Here's how the part is built. I have some questions about the finished solid (model axes, mm). Face numbers are marked on the shaded views. A direction names the side the tool comes from. Round coordinates to 2 decimals unless told otherwise and drop trailing zeros. Order: outer loops, then holes, each group sorted by start corner. A loop starts at its lowest first (then second) coordinate and runs counter-clockwise, first axis right, second up. Notation, with made-up numbers: (-24.75, 63.5) -> (19.25, 63.5) arc R18 ccw to (19.25, 71.5) -> close; hole circle Ø5 at (-32, 72). An arc over 180 degrees is marked (long way). One line per item, written item: value.
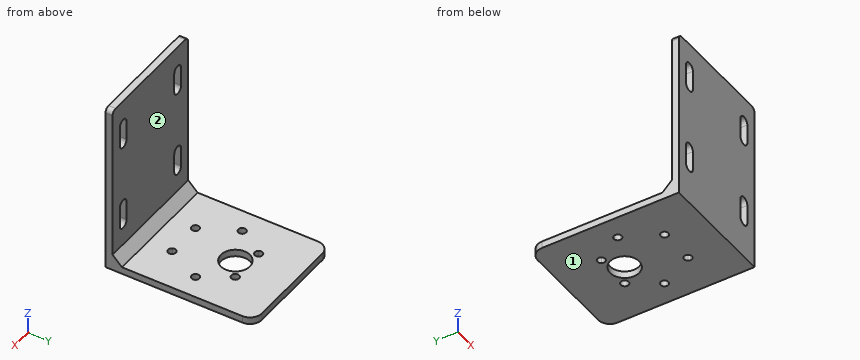
```python
from build123d import *

# Parameters (mm, degrees)
EXTRUDE_2_DEPTH     = 3
SKETCH_2_W          = 50
SKETCH_2_H          = 3
EXTRUDE_3_DEPTH     = 3
SKETCH_3_W          = 50
SKETCH_3_H          = 3
EXTRUDE_5_DEPTH     = 70
CUT_EXTRUDE_1_DEPTH = 98.744565066
FILLET_1_R          = 5
FILLET_2_R          = 2
SKETCH_5_W          = 4
SKETCH_5_H          = 4
EXTRUDE_6_DEPTH     = 4
SKETCH_6_W          = 4
SKETCH_6_H          = 4
EXTRUDE_7_DEPTH     = 46
CUT_EXTRUDE_2_DEPTH = 95.435162943


with BuildPart() as part:
    # 草图1 → 凸台-拉伸2 (new body)
    with BuildSketch(Plane.XY):
        with BuildLine():
            Line((25, 6), (25, 30))
            Line((25, 30), (-25, 30))
            Line((-25, 30), (-25, 6))
            Line((-25, 6), (-16.431676725, 6))
            ThreePointArc((-16.431676725, 6), (0, 16), (16.431676725, 6))
            Line((16.431676725, 6), (25, 6))
        make_face()
        with BuildLine():
            Line((25, -30), (25, -1))
            Line((25, -1), (18.439088915, -1))
            ThreePointArc((18.439088915, -1), (18.484765956, -1.749381895), (18.5, -2.5))
            ThreePointArc((18.5, -2.5), (-4.374013065, -20.475483574), (-16.431676725, 6))
            Line((-16.431676725, 6), (-25, 6))
            Line((-25, 6), (-25, -30))
            Line((-25, -30), (25, -30))
        make_face()
        with BuildLine():
            Line((25, -1), (25, 6))
            Line((25, 6), (16.431676725, 6))
            ThreePointArc((16.431676725, 6), (17.783210455, 2.599747633), (18.439088915, -1))
            Line((18.439088915, -1), (25, -1))
        make_face()
        with BuildLine():
            ThreePointArc((18.5, -2.5), (18.484765956, -1.749381895), (18.439088915, -1))
            Line((18.439088915, -1), (17.077248621, -1))
            ThreePointArc((17.077248621, -1), (16.619172939, -2.1409717), (15.499289324, -2.648426564))
            ThreePointArc((15.499289324, -2.648426564), (13.783292906, -9.590192993), (9.133777755, -15.022943101))
            ThreePointArc((9.133777755, -15.022943101), (9.324554056, -15.446200161), (9.389869855, -15.905847832))
            ThreePointArc((9.389869855, -15.905847832), (8.134145395, -17.508048443), (6.278297978, -16.671555119))
            ThreePointArc((6.278297978, -16.671555119), (0, -18), (-6.278297978, -16.671555119))
            ThreePointArc((-6.278297978, -16.671555119), (-8.564869855, -17.334789748), (-9.133777755, -15.022943101))
            ThreePointArc((-9.133777755, -15.022943101), (-13.783292906, -9.590192993), (-15.499289324, -2.648426564))
            ThreePointArc((-15.499289324, -2.648426564), (-17.069504119, -0.840322581), (-15.18038717, 0.631428645))
            ThreePointArc((-15.18038717, 0.631428645), (-14.324684332, 3.420592774), (-12.961481397, 6))
            Line((-12.961481397, 6), (-16.431676725, 6))
            ThreePointArc((-16.431676725, 6), (-4.374013065, -20.475483574), (18.5, -2.5))
        make_face()
        with BuildLine():
            Line((12.961481397, 6), (16.431676725, 6))
            ThreePointArc((16.431676725, 6), (0, 16), (-16.431676725, 6))
            Line((-16.431676725, 6), (-12.961481397, 6))
            ThreePointArc((-12.961481397, 6), (-11.229253628, 8.184281115), (-9.133777755, 10.022943101))
            ThreePointArc((-9.133777755, 10.022943101), (-8.564869855, 12.334789748), (-6.278297978, 11.671555119))
            ThreePointArc((-6.278297978, 11.671555119), (0, 13), (6.278297978, 11.671555119))
            ThreePointArc((6.278297978, 11.671555119), (8.134145395, 12.508048443), (9.389869855, 10.905847832))
            ThreePointArc((9.389869855, 10.905847832), (9.324554056, 10.446200161), (9.133777755, 10.022943101))
            ThreePointArc((9.133777755, 10.022943101), (11.229253628, 8.184281115), (12.961481397, 6))
        make_face()
        with BuildLine():
            ThreePointArc((15.18038717, 0.631428645), (14.324684332, 3.420592774), (12.961481397, 6))
            Line((12.961481397, 6), (6.15, 6))
            ThreePointArc((6.15, 6), (0, -0.15), (-6.15, 6))
            Line((-6.15, 6), (-12.961481397, 6))
            ThreePointArc((-12.961481397, 6), (-14.324684332, 3.420592774), (-15.18038717, 0.631428645))
            ThreePointArc((-15.18038717, 0.631428645), (-14.176284714, 0.075913242), (-13.777248621, -1))
            ThreePointArc((-13.777248621, -1), (-14.286276921, -2.191924318), (-15.499289324, -2.648426564))
            ThreePointArc((-15.499289324, -2.648426564), (-13.783292906, -9.590192993), (-9.133777755, -15.022943101))
            ThreePointArc((-9.133777755, -15.022943101), (-7.280222183, -14.321163631), (-6.089869855, -15.905847832))
            ThreePointArc((-6.089869855, -15.905847832), (-6.137669243, -16.300123373), (-6.278297978, -16.671555119))
            ThreePointArc((-6.278297978, -16.671555119), (0, -18), (6.278297978, -16.671555119))
            ThreePointArc((6.278297978, -16.671555119), (6.914869855, -14.476905916), (9.133777755, -15.022943101))
            ThreePointArc((9.133777755, -15.022943101), (13.783292906, -9.590192993), (15.499289324, -2.648426564))
            ThreePointArc((15.499289324, -2.648426564), (13.784993122, -1.159677419), (15.18038717, 0.631428645))
        make_face()
        with BuildLine():
            Line((6.15, 6), (12.961481397, 6))
            ThreePointArc((12.961481397, 6), (11.229253628, 8.184281115), (9.133777755, 10.022943101))
            ThreePointArc((9.133777755, 10.022943101), (6.914869855, 9.476905916), (6.278297978, 11.671555119))
            ThreePointArc((6.278297978, 11.671555119), (0, 13), (-6.278297978, 11.671555119))
            ThreePointArc((-6.278297978, 11.671555119), (-6.137669243, 11.300123373), (-6.089869855, 10.905847832))
            ThreePointArc((-6.089869855, 10.905847832), (-7.280222183, 9.321163631), (-9.133777755, 10.022943101))
            ThreePointArc((-9.133777755, 10.022943101), (-11.229253628, 8.184281115), (-12.961481397, 6))
            Line((-12.961481397, 6), (-6.15, 6))
            ThreePointArc((-6.15, 6), (0, 12.15), (6.15, 6))
        make_face()
        with BuildLine():
            ThreePointArc((18.439088915, -1), (17.783210455, 2.599747633), (16.431676725, 6))
            Line((16.431676725, 6), (12.961481397, 6))
            ThreePointArc((12.961481397, 6), (14.324684332, 3.420592774), (15.18038717, 0.631428645))
            ThreePointArc((15.18038717, 0.631428645), (16.503161862, 0.250963907), (17.077248621, -1))
            Line((17.077248621, -1), (18.439088915, -1))
        make_face()
    extrude(amount=EXTRUDE_2_DEPTH)

    # 草图2 → 凸台-拉伸3 (add)
    with BuildSketch(Plane.XZ.offset(30)):
        with Locations((0, 1.5)):
            Rectangle(SKETCH_2_W, SKETCH_2_H)
    extrude(amount=EXTRUDE_3_DEPTH)

    # 草图3 → 凸台-拉伸5 (add)
    with BuildSketch(Plane.XY.offset(3)):
        with Locations((0, -31.5)):
            Rectangle(SKETCH_3_W, SKETCH_3_H)
    extrude(amount=EXTRUDE_5_DEPTH)

    # 草图4 → 切除-拉伸1 (cut, through all)
    with BuildSketch(Plane(origin=(0, -30, 0), x_dir=(1, 0, 0), z_dir=(0, 1, 0))):
        with BuildLine():
            Line((-15.75, -53.85), (-15.75, -62.15))
            ThreePointArc((-15.75, -62.15), (-18, -64.4), (-20.25, -62.15))
            Line((-20.25, -62.15), (-20.25, -53.85))
            ThreePointArc((-20.25, -53.85), (-18, -51.6), (-15.75, -53.85))
        make_face()
        with BuildLine():
            Line((15.75, -53.85), (15.75, -62.15))
            ThreePointArc((15.75, -62.15), (18, -64.4), (20.25, -62.15))
            Line((20.25, -62.15), (20.25, -53.85))
            ThreePointArc((20.25, -53.85), (18, -51.6), (15.75, -53.85))
        make_face()
        with BuildLine():
            Line((-15.75, -16.85), (-15.75, -25.15))
            ThreePointArc((-15.75, -25.15), (-18, -27.4), (-20.25, -25.15))
            Line((-20.25, -25.15), (-20.25, -16.85))
            ThreePointArc((-20.25, -16.85), (-18, -14.6), (-15.75, -16.85))
        make_face()
        with BuildLine():
            Line((15.75, -16.85), (15.75, -25.15))
            ThreePointArc((15.75, -25.15), (18, -27.4), (20.25, -25.15))
            Line((20.25, -25.15), (20.25, -16.85))
            ThreePointArc((20.25, -16.85), (18, -14.6), (15.75, -16.85))
        make_face()
    extrude(amount=-CUT_EXTRUDE_1_DEPTH, mode=Mode.SUBTRACT)

    # 圆角1
    fillet_1_edges = [part.edges().sort_by_distance(p)[0] for p in [
        (-25, 30, 1.5),
        (25, 30, 1.5),
    ]]
    fillet(fillet_1_edges, radius=FILLET_1_R)

    # 圆角2
    fillet_2_edges = [part.edges().sort_by_distance(p)[0] for p in [
        (25, -31.5, 73),
        (-25, -31.5, 73),
    ]]
    fillet(fillet_2_edges, radius=FILLET_2_R)

    # 草图5 → 凸台-拉伸6 (add)
    with BuildSketch(Plane(origin=(0, -30, 0), x_dir=(1, 0, 0), z_dir=(0, 1, 0))):
        with Locations((23, -5)):
            Rectangle(SKETCH_5_W, SKETCH_5_H)
    extrude(amount=EXTRUDE_6_DEPTH)

    # 草图6 → 凸台-拉伸7 (add)
    with BuildSketch(Plane.ZY.offset(-21)):
        with Locations((5, -28)):
            Rectangle(SKETCH_6_W, SKETCH_6_H)
    extrude(amount=EXTRUDE_7_DEPTH)

    # 草图7 → 切除-拉伸2 (cut, through all)
    with BuildSketch(Plane(origin=(25, 0, 0), x_dir=(0, 0, -1), z_dir=(1, 0, 0))):
        Polygon((-7, -30), (-7, -26), (-3, -26), align=None)
    extrude(amount=-CUT_EXTRUDE_2_DEPTH, mode=Mode.SUBTRACT)


solid = part.part
```
Q1. Which directions (+Z, -Z, +X, -X, +Y, -Y) give clear straight access to the entire face, cutting with the end or side of a thin tool? Please do the marked faces 1 and 2.
Answers:
face 1: -Z, +X, -X, +Y, -Y
face 2: +Z, +X, -X, +Y
Q2. I need wall thicknesses on line 1 along Y through (x, z) = (0, 2.25); line 2 along Z through (x, y) = (14, 20.5); line 3 along Y through (x, z) = (10, 42.5). Which ranges of each line are inside material? Lowest first, please.
Answers:
line 1: -33 to -0.15, 12.15 to 30
line 2: 0 to 3
line 3: -33 to -30
Q3. I want a section at D-D on x = -18. Write out the boundary of the cut face in (y, z), then the cut area to 3 significant figures.
Answers:
outline: (-33, 0) -> (30, 0) -> (30, 3) -> (-26, 3) -> (-30, 7) -> (-30, 14.6) -> (-33, 14.6) -> close; (-33, 27.4) -> (-30, 27.4) -> (-30, 51.6) -> (-33, 51.6) -> close; (-33, 64.4) -> (-30, 64.4) -> (-30, 73) -> (-33, 73) -> close
area: 330 mm2
Q4. I want a section at A-A on x = 0. Write out the boundary of the cut face in (y, z).
Answers:
outline: (-33, 0) -> (-0.15, 0) -> (-0.15, 3) -> (-26, 3) -> (-30, 7) -> (-30, 73) -> (-33, 73) -> close; (12.15, 0) -> (30, 0) -> (30, 3) -> (12.15, 3) -> close
Q5. I want a section at B-B on z = 19. Write out the boundary of the cut face in (x, y), then the cut area to 3 significant figures.
Answers:
outline: (-25, -33) -> (-20.25, -33) -> (-20.25, -30) -> (-25, -30) -> close; (-15.75, -33) -> (15.75, -33) -> (15.75, -30) -> (-15.75, -30) -> close; (20.25, -33) -> (25, -33) -> (25, -30) -> (20.25, -30) -> close
area: 123 mm2
Q6. I want a section at C-C on y = 6. Write out the boundary of the cut face in (x, z), then the cut area to 3 significant figures.
Answers:
outline: (-25, 0) -> (-6.15, 0) -> (-6.15, 3) -> (-25, 3) -> close; (6.15, 0) -> (25, 0) -> (25, 3) -> (6.15, 3) -> close
area: 113 mm2
Q7. For P1, Ø25, axis at x = -5.5, y = -7, coming from the +Z side, with a flat end and sliding along its axis, tell me the tip position at first contact or that it passes through.
Answers:
P1: z = 3
